from build123d import *

# Parameters (mm, degrees)
SKETCH1_W           = 58
SKETCH1_H           = 40
BOSS_EXTRUDE1_DEPTH = 1
SKETCH2_W           = 6.25
SKETCH2_H           = 12.5
BOSS_EXTRUDE2_DEPTH = 5
CHAMFER1_SIZE       = 1
SKETCH3_W           = 9.2
SKETCH3_H           = 5
BOSS_EXTRUDE3_DEPTH = 3
SKETCH4_W           = 5
SKETCH4_H           = 6.6
BOSS_EXTRUDE4_DEPTH = 4
SKETCH5_R           = 1.6
CUT_EXTRUDE1_DEPTH  = 6


with BuildPart() as part:
    # Sketch1 → Boss-Extrude1 (new body)
    with BuildSketch(Plane(origin=(0, 0, 0), x_dir=(1, 0, 0), z_dir=(0, 1, 0))):
        Rectangle(SKETCH1_W, SKETCH1_H)
    extrude(amount=BOSS_EXTRUDE1_DEPTH)

    # Sketch2 → Boss-Extrude2 (add)
    with BuildSketch(Plane(origin=(0, 1, 0), x_dir=(1, 0, 0), z_dir=(0, 1, 0))):
        with Locations((29.475, 0)):
            Rectangle(SKETCH2_W, SKETCH2_H)
    extrude(amount=BOSS_EXTRUDE2_DEPTH)

    # Chamfer1
    chamfer1_edges = [part.edges().sort_by_distance(p)[0] for p in [
        (30.8, 1, -6.25),
    ]]
    chamfer(chamfer1_edges, length=CHAMFER1_SIZE)

    # Sketch3 → Boss-Extrude3 (add)
    with BuildSketch(Plane(origin=(0, 1, 0), x_dir=(1, 0, 0), z_dir=(0, 1, 0))):
        with Locations((-2.9, 18.5)):
            Rectangle(SKETCH3_W, SKETCH3_H)
    extrude(amount=BOSS_EXTRUDE3_DEPTH)

    # Sketch4 → Boss-Extrude4 (add)
    with BuildSketch(Plane.XZ):
        with Locations((-25.5, 8.7)):
            Rectangle(SKETCH4_W, SKETCH4_H)
        with Locations((-25.5, -8.9)):
            Rectangle(SKETCH4_W, SKETCH4_H)
        with Locations((20, 8.7)):
            Rectangle(SKETCH4_W, SKETCH4_H)
        with Locations((20, -8.9)):
            Rectangle(SKETCH4_W, SKETCH4_H)
    extrude(amount=BOSS_EXTRUDE4_DEPTH)

    # Sketch5 → Cut-Extrude1 (cut, through all)
    with BuildSketch(Plane(origin=(0, 1, 0), x_dir=(1, 0, 0), z_dir=(0, 1, 0))):
        with Locations((-23.25, 17.5)):
            Circle(SKETCH5_R)
        with Locations((-23.25, -17.5)):
            Circle(SKETCH5_R)
        with Locations((23.25, -17.5)):
            Circle(SKETCH5_R)
        with Locations((23.25, 17.5)):
            Circle(SKETCH5_R)
    extrude(amount=-CUT_EXTRUDE1_DEPTH, mode=Mode.SUBTRACT)


solid = part.part
Source: CAD feature listing. Evaluate the final solid. Frame: model axes, mm. A direction names the side the tool comes from. Coordinates: 2 decimals unless noted, no trailing zeros. Loops run counter-clockwise (first coordinate to the right, second up) from the corner with the lowest first, then second, coordinate; pieces in that order, holes last. Notation, with made-up numbers: (56, -16.5) -> (104, -16.5) arc R31 ccw to (104, 9.5) -> close; hole circle Ø1 at (-33.75, -15.75). An arc over 180 degrees is marked (long way). Answer in a Markdown table with one row per item. Add a question column.
Q1. Section B-B on x = 23.25. Return the cut outline in (y, z).
Q2. Reachability of faces 4 (the face through (-26, -2, 5.4)), 5 (the face through (-7.5, 2, -18)), 6 (the face through (-26, -2, -12.2)), 7 (the face through (17.5, -2, 9)), 8 (the face through (31, 1, 0)) from +Z, -Z, +X, -X, +Y, -Y: full face, straight path, thin tool, end or side. Return the list, or none.
Q3. Section A-A on z = -17.5. Return the cut outline in (x, y).
Q4. Pull-direction query (X, two-part tool) for faces 1 (the face through (-28, -2, -9)), 2 (the face through (20, -2, 12)), 3 (the face through (-23.458, 0.507, -19.086)); classes: pulls with the +X half, pulls with the -X half, needs draft (parallel to the pull), parting line crosses it, or undercut.
Q5. Section C-C on z = -1. Return the cut outline in (x, y), and give its area (4 significant figures).
Q6. Section D-D on z = 17.5. Return the cut outline in (x, y), and give its area (3 significant figures).
Q7. Contact query for flat-ended pins moving along their axis: pin 1 Ø4 at (x, z) = (-4.5, -6) entering from -Y; pin 2 Ø0.9 at (y, z) = (2.5, -19) entering from -X; pin 3 Ø3 at (y, z) = (-2, -8) entering from -X; pin 4 Ø4.5 at (y, z) = (-2, 7) entering from -X. Output: stop coordinate, or through.
Q8. Ray query, line 1 along X through (y, z) = (0.3, -17.5); line 2 along Z through (x, y) = (23.25, 0.5); line 3 along Z through (x, y) = (19.5, -3). Return the intervals inside material, ascending.
Computed values:
| question | item | result |
|---|---|---|
| 1 | outline | (0, -20) -> (1, -20) -> (1, -19.1) -> (0, -19.1) -> close; (0, -15.9) -> (1, -15.9) -> (1, 15.9) -> (0, 15.9) -> close; (0, 19.1) -> (1, 19.1) -> (1, 20) -> (0, 20) -> close |
| 2 | face 4 | +X, -X, -Y |
| 2 | face 5 | +Z, -Z, -X, +Y |
| 2 | face 6 | -Z, +X, -X, -Y |
| 2 | face 7 | +Z, -Z, -Y |
| 2 | face 8 | +Z, -Z, +X, -Y |
| 3 | outline | (-29, 0) -> (-24.85, 0) -> (-24.85, 1) -> (-29, 1) -> close; (-21.65, 0) -> (21.65, 0) -> (21.65, 1) -> (1.7, 1) -> (1.7, 4) -> (-7.5, 4) -> (-7.5, 1) -> (-21.65, 1) -> close; (24.85, 0) -> (29, 0) -> (29, 1) -> (24.85, 1) -> close |
| 4 | face 1 | pulls with the -X half |
| 4 | face 2 | needs draft |
| 4 | face 3 | undercut |
| 5 | outline | (-29, 0) -> (29, 0) -> (29, 1) -> (32.6, 1) -> (32.6, 6) -> (26.35, 6) -> (26.35, 1) -> (-29, 1) -> close |
| 5 | area | 89.25 mm^2 |
| 6 | outline | (-29, 0) -> (-24.85, 0) -> (-24.85, 1) -> (-29, 1) -> close; (-21.65, 0) -> (21.65, 0) -> (21.65, 1) -> (-21.65, 1) -> close; (24.85, 0) -> (29, 0) -> (29, 1) -> (24.85, 1) -> close |
| 6 | area | 51.6 mm^2 |
| 7 | pin 1 | stops at y = 0 |
| 7 | pin 2 | stops at x = -7.5 |
| 7 | pin 3 | stops at x = -28 |
| 7 | pin 4 | stops at x = -29 |
| 8 | line 1 | x = -29 to -24.85, -21.65 to 21.65, 24.85 to 29 |
| 8 | line 2 | z = -20 to -19.1, -15.9 to 15.9, 19.1 to 20 |
| 8 | line 3 | z = -12.2 to -5.6, 5.4 to 12 |
